Design review of the part built by this model. Coordinates are the model's own, in mm. Face numbers are marked on the shaded views. A direction names the side the tool comes from. Round coordinates to 2 decimals unless told otherwise and drop trailing zeros. Write each loop counter-clockwise with the first axis right and the second up, starting at its lowest first coordinate (ties: lowest second). Pieces come first, ordered by that corner, then holes.
from build123d import *

# Parameters (mm, degrees)
BOSS_EXTRUDE2_DEPTH       = 36
CUT_EXTRUDE1_DEPTH        = 43
FILLET1_R                 = 6
CUT_EXTRUDE2_DEPTH        = 43
FILLET2_R                 = 6
F_6_0MM_DOWEL_HOLE1_D     = 6
F_6_0MM_DOWEL_HOLE1_DEPTH = 6
F_6_0MM_DOWEL_HOLE1_TIP   = 1.802581857
SKETCH23_W                = 20
SKETCH23_H                = 20
CUT_EXTRUDE4_DEPTH        = 8
CUT_EXTRUDE5_DEPTH        = 12.0000001


with BuildPart() as part:
    # Sketch1 → Boss-Extrude2 (new body)
    with BuildSketch(Plane.XY):
        with BuildLine():
            Line((50, -27), (79, -27))
            Line((79, -27), (82, -38))
            Line((82, -38), (-82, -38))
            Line((-82, -38), (-79, -27))
            Line((-79, -27), (-50, -27))
            Line((-50, -27), (-50, 16))
            Line((-50, 16), (-22, 16))
            Line((-22, 16), (-22, 3))
            Line((-22, 3), (-19, 3))
            Line((-19, 3), (-19, 0))
            ThreePointArc((-19, 0), (0, -19), (19, 0))
            Line((19, 0), (19, 3))
            Line((19, 3), (22, 3))
            Line((22, 3), (22, 16))
            Line((22, 16), (50, 16))
            Line((50, 16), (50, -27))
        make_face()
    extrude(amount=BOSS_EXTRUDE2_DEPTH)

    # Sketch11 → Cut-Extrude1 (cut)
    with BuildSketch(Plane(origin=(0, 16, 0), x_dir=(1, 0, 0), z_dir=(0, 1, 0))):
        with BuildLine():
            Line((-50, 0), (-50, -36))
            Line((-50, -36), (-37.523326079, -36))
            ThreePointArc((-37.523326079, -36), (-43.785692077, -18), (-37.523326079, 0))
            Line((-37.523326079, 0), (-50, 0))
        make_face()
    extrude(amount=-CUT_EXTRUDE1_DEPTH, mode=Mode.SUBTRACT)

    # Fillet1
    fillet1_edges = [part.edges().sort_by_distance(p)[0] for p in [
        (-43.785692077, -27, 18),
    ]]
    fillet(fillet1_edges, radius=FILLET1_R)

    # Sketch12 → Cut-Extrude2 (cut)
    with BuildSketch(Plane(origin=(0, 16, 0), x_dir=(1, 0, 0), z_dir=(0, 1, 0))):
        with BuildLine():
            Line((37.994971795, 0), (50, 0))
            Line((50, 0), (50, -36))
            Line((50, -36), (37.994971795, -36))
            ThreePointArc((37.994971795, -36), (44.257337793, -18), (37.994971795, 0))
        make_face()
    extrude(amount=-CUT_EXTRUDE2_DEPTH, mode=Mode.SUBTRACT)

    # Fillet2
    fillet2_edges = [part.edges().sort_by_distance(p)[0] for p in [
        (44.257337793, -27, 18),
    ]]
    fillet(fillet2_edges, radius=FILLET2_R)

    # Ø6.0mm Dowel Hole1
    with Locations(Plane(origin=(0, -19, 18), x_dir=(1, 0, 0), z_dir=(0, 1, 0))):
        with Locations((0, 0)):
            Hole(F_6_0MM_DOWEL_HOLE1_D / 2, depth=F_6_0MM_DOWEL_HOLE1_DEPTH)
            with Locations((0, 0, -(F_6_0MM_DOWEL_HOLE1_DEPTH + F_6_0MM_DOWEL_HOLE1_TIP / 2))):  # 118° drill point
                Cone(0, F_6_0MM_DOWEL_HOLE1_D / 2, F_6_0MM_DOWEL_HOLE1_TIP, mode=Mode.SUBTRACT)

    # Sketch19 → Ø6.0mm Dowel Hole3 (revolve, cut)
    with BuildSketch(Plane(origin=(-31, 16, 18), x_dir=(0, 0, 1), z_dir=(1, 0, 0))):
        Polygon((0, 0), (0, 48.703872786), (4.5, 46), (4.5, 0), align=None)
    f_6_0mm_dowel_hole3 = revolve(axis=Axis((-31, 22.35, 18), (0, -1, 0)), mode=Mode.SUBTRACT)

    # Sketch23 → Cut-Extrude4 (cut)
    with BuildSketch(Plane.XZ.offset(38)):
        with Locations((-31, 18)):
            Rectangle(SKETCH23_W, SKETCH23_H)
    cut_extrude4 = extrude(amount=-CUT_EXTRUDE4_DEPTH, mode=Mode.SUBTRACT)

    # Mirror1: Ø6.0mm Dowel Hole3, Cut-Extrude4 across plane
    add(f_6_0mm_dowel_hole3.mirror(Plane(origin=(0, 0, 0), x_dir=(0, 0, 1), z_dir=(1, 0, 0))), mode=Mode.SUBTRACT)
    add(cut_extrude4.mirror(Plane(origin=(0, 0, 0), x_dir=(0, 0, 1), z_dir=(1, 0, 0))), mode=Mode.SUBTRACT)

    # Sketch25 → Cut-Extrude5 (cut, through all)
    with BuildSketch(Plane(origin=(0, -27, 0), x_dir=(1, 0, 0), z_dir=(0, 1, 0))):
        with BuildLine():
            Line((-67.5, -13.5), (-60.5, -13.5))
            ThreePointArc((-60.5, -13.5), (-56, -18), (-60.5, -22.5))
            Line((-60.5, -22.5), (-67.5, -22.5))
            ThreePointArc((-67.5, -22.5), (-72, -18), (-67.5, -13.5))
        make_face()
    cut_extrude5 = extrude(amount=-CUT_EXTRUDE5_DEPTH, mode=Mode.SUBTRACT)

    # Mirror2: Cut-Extrude5 across plane
    add(cut_extrude5.mirror(Plane(origin=(0, 0, 0), x_dir=(0, 0, 1), z_dir=(1, 0, 0))), mode=Mode.SUBTRACT)


solid = part.part
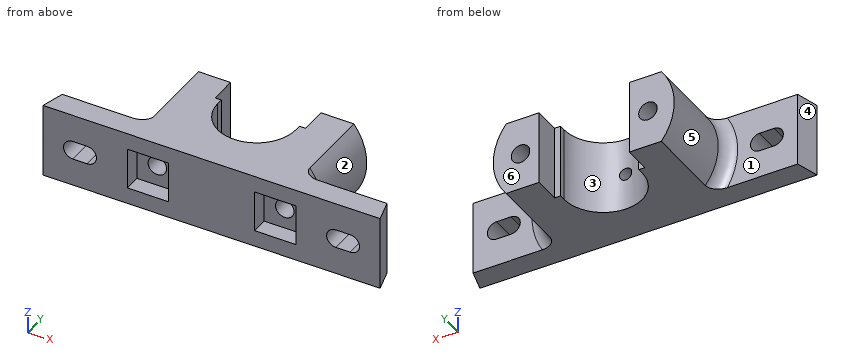
1) Add section B-B on x = 31. State the section outline as (y, z) points, and give its area (3 significant figures).
2) For P1, Ø16, axis at x = -30, z = 22.5, coming from the -Y side; P2, Ø2.5, axis at y = 2, z = 12, coming from the +X side; P3, Ø12, axis at x = 3.5, z = 24.5, coming from the +Y side; P4, Ø10.5, axis at y = 9.5, z = 9.5, coming from the -X side, all flat-tipped, find the tip position at first contact; note any pin that passes through.
3) Add section C-C on x = -69.5. State the section outline as (y, z) points.
4) For line 1 along X through (y, z) = (-21, 18); line 2 along Z through (x, y) = (-31, -14); line 3 along X through (y, z) = (-3.5, 18), list the stretches that pass through material, from the lowest coordinate up.
5) For the marked faces 5 and 6, list the 3-axis set-ups (+Z, -Z, +X, -X, +Y, -Y) from which the entire face can be reached by the end or side of a thin tool; tool diameter is ignored.
6) The part is to be moulded in two halves that separate along X. For the marked faces 1, 2, 3 and 4, say which applies: pulls with the +X half, pulls with the -X half, needs draft (parallel to the pull), parting line crosses it, or undercut.
7) Add section A-A on y = -14. State the section outline as (x, z) points.
Computed:
1. outline: (-38, 0) - (16, 0) - (16, 13.5) - (-30, 13.5) - (-30, 8) - (-38, 8) - close; (-38, 28) - (-30, 28) - (-30, 22.5) - (16, 22.5) - (16, 36) - (-38, 36) - close
1. area: 1,370 mm2
2. P1: stops at y = -38
2. P2: stops at x = 43.87
2. P3: stops at y = -16.45
2. P4: stops at x = -43.6
3. outline: (-38, 0) - (-27, 0) - (-27, 13.97) - (-38, 13.97) - close; (-38, 22.03) - (-27, 22.03) - (-27, 36) - (-38, 36) - close
4. line 1: x = -43.79 to -35.5, -26.5 to -3, 3 to 26.5, 35.5 to 44.26
4. line 2: z = 0 to 13.5, 22.5 to 36
4. line 3: x = -43.79 to -35.5, -26.5 to -18.67, 18.67 to 26.5, 35.5 to 44.26
5. face 5: -X, +Y
5. face 6: +Z, -Z, +X, -X, +Y
6. face 1: needs draft
6. face 2: pulls with the +X half
6. face 3: undercut
6. face 4: pulls with the -X half
7. outline: (-37.52, 0) - (-12.85, 0) - (-12.85, 36) - (-37.52, 36) arc R29 ccw to start; (12.85, 0) - (37.99, 0) arc R29 ccw to (37.99, 36) - (12.85, 36) - close; hole circle Ø9 at (-31, 18); hole circle Ø9 at (31, 18)
